The model under review builds one solid part; all positions refer to its coordinate system, in mm. Round coordinates to 2 decimals unless told otherwise and drop trailing zeros. Loops run counter-clockwise (first coordinate to the right, second up) from the corner with the lowest first, then second, coordinate; pieces in that order, holes last. Notation, with made-up numbers: (21.5, -23) -> (60.5, -23) arc R17 ccw to (60.5, -14) -> close; hole circle Ø2 at (55.25, 3.5). An arc over 180 degrees is marked (long way). Write each question's results on one line, items separated by ' | '. Start each with the question number.
Item 1: We need section D-D (z = -32.5). Give the boundary of the cut face in (x, y), and give its area (3 significant figures).
Item 2: We need section C-C (x = -32.5). Give the boundary of the cut face in (y, z).
Item 3: Clearance check with flat-ended pins moving along their axes: pin 1 Ø6.5 at (x, z) = (31, -1) entering from +Y; pin 2 Ø2 at (y, z) = (2, -12.5) entering from -X; pin 3 Ø5 at (x, z) = (0, -32.5) entering from +Y; pin 4 Ø2 at (y, z) = (2.5, -2) entering from -X. State where each tip first meets the part, or that it passes through.
Item 4: We need section B-B (z = 0). Give the boundary of the cut face in (x, y), and give its area (3 significant figures).
Item 5: For L1, parallel to X at y = 4.1, z = 0; L2, parallel to X at y = 4.1, z = -24.5; L3, parallel to Z at x = 30.5, y = 1.65, list the stretches that pass through material, from the lowest coordinate up. Write a range as from..to.
Item 6: We need section A-A (x = 0). Give the boundary of the cut face in (y, z).
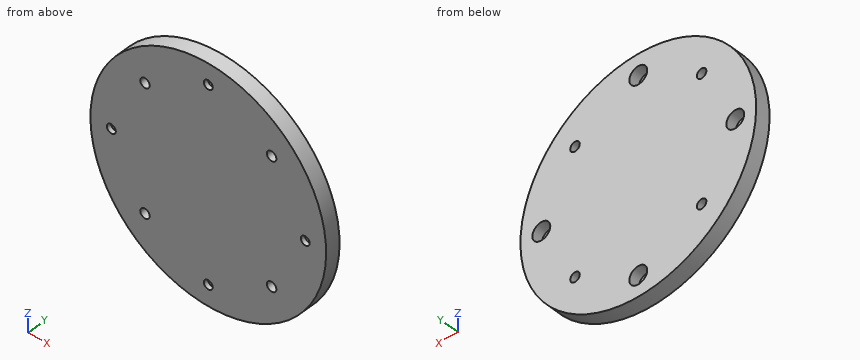
from build123d import *

# Parameters (mm, degrees)
SKETCH_1_R               = 39.5
EXTRUDE_1_DEPTH          = 5
CUT_EXTRUDE_1_DEPTH      = 57.084757288
CUT_EXTRUDE_1_DEPTH_BACK = 57.084757288
SKETCH_2_R               = 1.5
SKETCH_3_R               = 3
CUT_EXTRUDE_2_DEPTH      = 3.5
SKETCH_5_R               = 1.6
CUT_EXTRUDE_3_DEPTH      = 57.084757288


with BuildPart() as part:
    # 草图1 → 凸台-拉伸1 (new body)
    with BuildSketch(Plane(origin=(0, 0, 0), x_dir=(1, 0, 0), z_dir=(0, 1, 0))):
        with Locations(Location((0, 0, 0), (0, 0, 270))):
            Circle(SKETCH_1_R)
    extrude(amount=EXTRUDE_1_DEPTH)

    # 草图2 → 切除-拉伸1 (cut, two sides: drawn at the far end of the back side and taken through both)
    with BuildSketch(Plane(origin=(0, 5, 0), x_dir=(1, 0, 0), z_dir=(0, 1, 0)).offset(-CUT_EXTRUDE_1_DEPTH_BACK)):
        with Locations(Location((0, 32.5, 0), (0, 0, 270))):
            Circle(SKETCH_2_R)
        with Locations(Location((32.5, 0, 0), (0, 0, 270))):
            Circle(SKETCH_2_R)
        with Locations(Location((0, -32.5, 0), (0, 0, 270))):
            Circle(SKETCH_2_R)
        with Locations(Location((-32.5, 0, 0), (0, 0, 270))):
            Circle(SKETCH_2_R)
    extrude(amount=CUT_EXTRUDE_1_DEPTH + CUT_EXTRUDE_1_DEPTH_BACK, mode=Mode.SUBTRACT)

    # 草图3 → 切除-拉伸2 (cut)
    with BuildSketch(Plane(origin=(0, 5, 0), x_dir=(1, 0, 0), z_dir=(0, 1, 0))):
        with Locations(Location((-32.5, 0, 0), (0, 0, 270))):
            Circle(SKETCH_3_R)
        with Locations(Location((0, -32.5, 0), (0, 0, 270))):
            Circle(SKETCH_3_R)
        with Locations(Location((32.5, 0, 0), (0, 0, 270))):
            Circle(SKETCH_3_R)
        with Locations(Location((0, 32.5, 0), (0, 0, 270))):
            Circle(SKETCH_3_R)
    extrude(amount=-CUT_EXTRUDE_2_DEPTH, mode=Mode.SUBTRACT)

    # 草图5 → 切除-拉伸3 (cut, through all)
    with BuildSketch(Plane.XZ):
        with Locations(Location((21.213203436, 21.213203436, 0), (0, 0, 270))):
            Circle(SKETCH_5_R)
        with Locations(Location((21.213203436, -21.213203436, 0), (0, 0, 270))):
            Circle(SKETCH_5_R)
        with Locations(Location((-21.213203436, -21.213203436, 0), (0, 0, 270))):
            Circle(SKETCH_5_R)
        with Locations(Location((-21.213203436, 21.213203436, 0), (0, 0, 270))):
            Circle(SKETCH_5_R)
    extrude(amount=-CUT_EXTRUDE_3_DEPTH, mode=Mode.SUBTRACT)


solid = part.part
Here are the results:
1) outline: (-22.45, 0) -> (-1.5, 0) -> (-1.5, 1.5) -> (-3, 1.5) -> (-3, 5) -> (-22.45, 5) -> close; (1.5, 0) -> (22.45, 0) -> (22.45, 5) -> (3, 5) -> (3, 1.5) -> (1.5, 1.5) -> close | area: 199 mm2
2) outline: (0, -22.45) -> (5, -22.45) -> (5, -3) -> (1.5, -3) -> (1.5, -1.5) -> (0, -1.5) -> close; (0, 1.5) -> (1.5, 1.5) -> (1.5, 3) -> (5, 3) -> (5, 22.45) -> (0, 22.45) -> close
3) pin 1: stops at y = 5 | pin 2: stops at x = -37.79 | pin 3: stops at y = 1.5 | pin 4: stops at x = -39.49
4) outline: (-39.5, 0) -> (-34, 0) -> (-34, 1.5) -> (-35.5, 1.5) -> (-35.5, 5) -> (-39.5, 5) -> close; (-31, 0) -> (31, 0) -> (31, 1.5) -> (29.5, 1.5) -> (29.5, 5) -> (-29.5, 5) -> (-29.5, 1.5) -> (-31, 1.5) -> close; (34, 0) -> (39.5, 0) -> (39.5, 5) -> (35.5, 5) -> (35.5, 1.5) -> (34, 1.5) -> close | area: 344 mm2
5) L1: x = -39.5..-35.5, -29.5..29.5, 35.5..39.5 | L2: x = -30.98..30.98 | L3: z = -25.1..-2.24, 2.24..25.1
6) outline: (0, -39.5) -> (5, -39.5) -> (5, -35.5) -> (1.5, -35.5) -> (1.5, -34) -> (0, -34) -> close; (0, -31) -> (1.5, -31) -> (1.5, -29.5) -> (5, -29.5) -> (5, 29.5) -> (1.5, 29.5) -> (1.5, 31) -> (0, 31) -> close; (0, 34) -> (1.5, 34) -> (1.5, 35.5) -> (5, 35.5) -> (5, 39.5) -> (0, 39.5) -> close
